Geometry check sheet. Reference: the model listing, model coordinates, mm. A direction names the side the tool comes from. Coordinates: 2 decimals unless noted, no trailing zeros. Write each loop counter-clockwise with the first axis right and the second up, starting at its lowest first coordinate (ties: lowest second). Pieces come first, ordered by that corner, then holes. Notation, with made-up numbers: M 31.5,58 L 72.5,58 A24 ccw 72.5,75 Z; hole C 78,-11 d11. An arc over 180 degrees is marked long. Write item = value, one per line. Start each with the question number.
```python
from build123d import *

# Parameters (mm, degrees)
ESQUISSE3_R             = 35
BOSS_EXTRU_3_DEPTH      = 5
ESQUISSE4_R             = 2
ESQUISSE4_R_2           = 1.6
ENL_V_MAT_EXTRU_1_DEPTH = 161.669919512


with BuildPart() as part:
    # Esquisse3 → Boss.-Extru.3 (new body)
    with BuildSketch(Plane(origin=(0, 0, 0), x_dir=(1, 0, 0), z_dir=(0, 1, 0))):
        with BuildLine():
            Line((-115, -25), (-25, -25))
            Line((-25, -25), (-24.99494949, -24.500051021))
            ThreePointArc((-24.99494949, -24.500051021), (-34.998214236, 0.353553761), (-24.494897428, 25))
            Line((-24.494897428, 25), (-25, 25))
            Line((-25, 25), (-115, 25))
            Line((-115, 25), (-115, -25))
        make_face()
        Circle(ESQUISSE3_R)
        Polygon((-9.403186381, -33.713203436), (35.849364905, -112.092921435), (79.150635095, -87.092921435), (34.150635095, -9.150635095), align=None)
        with BuildLine():
            Line((-24.494897428, 25), (-24.99494949, -24.500051021))
            ThreePointArc((-24.99494949, -24.500051021), (-17.805293657, -30.132565736), (-9.403186381, -33.713203436))
            Line((-9.403186381, -33.713203436), (33.715141323, -9.396235714))
            ThreePointArc((33.715141323, -9.396235714), (34.677297662, -4.741837919), (35, 0))
            ThreePointArc((35, 0), (34.72342821, 4.391302011), (33.898083809, 8.713203436))
            Line((33.898083809, 8.713203436), (-8.720191833, 33.896286735))
            ThreePointArc((-8.720191833, 33.896286735), (-17.19292058, 30.486119496), (-24.494897428, 25))
        make_face()
        Circle(ESQUISSE3_R)
        Polygon((33.898083809, 8.713203436), (79.150635095, 87.092921435), (35.849364905, 112.092921435), (-9.150635095, 34.150635095), align=None)
        with BuildLine():
            ThreePointArc((33.898083809, 8.713203436), (17.805293657, 30.132565736), (-8.720191833, 33.896286735))
            Line((-8.720191833, 33.896286735), (33.898083809, 8.713203436))
        make_face()
    extrude(amount=BOSS_EXTRU_3_DEPTH)

    # Esquisse4 → Enlèv. mat.-Extru.1 (cut, through all)
    with BuildSketch(Plane(origin=(0, 5, 0), x_dir=(1, 0, 0), z_dir=(0, 1, 0))):
        with Locations(Location((-101.75, 20, 0), (0, 0, 270))):
            Circle(ESQUISSE4_R)
        with Locations(Location((-101.75, -20, 0), (0, 0, 270))):
            Circle(ESQUISSE4_R)
        with Locations(Location((33.554491924, -98.118084835, 0), (0, 0, 270))):
            Circle(ESQUISSE4_R)
        with Locations(Location((68.195508076, -78.118084835, 0), (0, 0, 270))):
            Circle(ESQUISSE4_R)
        with Locations(Location((68.195508076, 78.118084835, 0), (0, 0, 270))):
            Circle(ESQUISSE4_R)
        with Locations(Location((33.554491924, 98.118084835, 0), (0, 0, 270))):
            Circle(ESQUISSE4_R)
        with Locations(Location((-3.248264889, -30.973840175, 0), (0, 0, 270))):
            Circle(ESQUISSE4_R_2)
        with Locations(Location((15.051735111, -62.670369954, 0), (0, 0, 270))):
            Circle(ESQUISSE4_R_2)
        with Locations(Location((28.448264889, -12.673840175, 0), (0, 0, 270))):
            Circle(ESQUISSE4_R_2)
        with Locations(Location((46.748264889, -44.370369954, 0), (0, 0, 270))):
            Circle(ESQUISSE4_R_2)
        with Locations(Location((28.448264889, 12.673840175, 0), (0, 0, 270))):
            Circle(ESQUISSE4_R_2)
        with Locations(Location((46.748264889, 44.370369954, 0), (0, 0, 270))):
            Circle(ESQUISSE4_R_2)
        with Locations(Location((15.051735111, 62.670369954, 0), (0, 0, 270))):
            Circle(ESQUISSE4_R_2)
        with Locations(Location((-3.248264889, 30.973840175, 0), (0, 0, 270))):
            Circle(ESQUISSE4_R_2)
        with Locations(Location((-25.2, 18.3, 0), (0, 0, 270))):
            Circle(ESQUISSE4_R_2)
        with Locations(Location((-61.8, -18.3, 0), (0, 0, 270))):
            Circle(ESQUISSE4_R_2)
        with Locations(Location((-25.2, -18.3, 0), (0, 0, 270))):
            Circle(ESQUISSE4_R_2)
        with Locations(Location((-61.8, 18.3, 0), (0, 0, 270))):
            Circle(ESQUISSE4_R_2)
    extrude(amount=-ENL_V_MAT_EXTRU_1_DEPTH, mode=Mode.SUBTRACT)


solid = part.part
```
Q1. Cross-section at B-B on x = -85. Enter the section's corners in (y, z).
Q2. Set-up check for faces 1 (the face through (56.208, 2.465, -47.354)), 2 (the face through (-69, 2, -25)), 3 (the face through (-71, 2, 25)): record each of +Z, -Z, +X, -X, +Y, -Y from which the full face is reachable in a straight line by a thin tool's end or side.
Q3. Cross-section at C-C on z = -38. Enter the section's corners in (x, y), and give its area (3 significant figures).
Q4. Cross-section at A-A on y = 4.05. Count the separate pieces of the cut face and the enclosed holes in it, and give its area (3 significant figures).
Q5. Gauge pin test, flat ends, axial feed: pin 1 (6.5 mm diameter, centred on x = -101.75, z = -20, fed in from -Y); pin 2 (1 mm diameter, centred on y = 4, z = 64, fed in from +X); pin 3 (1 mm diameter, centred on y = 4, z = -56.5, fed in from -X). Record the tip position at first contact, or that the pin passes through.
Q6. Scan lines: L1, parallel to Z at x = -3, y = 2.35; L2, parallel to Z at x = 68, y = 1.35; L3, parallel to Z at x = -59, y = 1.5. Record each from-to range of solid material in increasing order.
Values found:
q1.outline = M 0,-25 L 5,-25 L 5,25 L 0,25 Z
q2.face_1 = +X, +Y, -Y
q2.face_2 = -Z, -X, +Y, -Y
q2.face_3 = +Z, -X, +Y, -Y
q3.outline = M -6.93,0 L 50.81,0 L 50.81,5 L -6.93,5 Z
q3.area = 289 mm²
q4.separate_pieces = 1
q4.enclosed_holes = 18
q4.area = 16,200 mm²
q5.pin_1 = 0
q5.pin_2 = 66.11
q5.pin_3 = 3.46
q6.L1 = -44.8 to -32.55, -29.39 to 29.39, 32.55 to 44.8
q6.L2 = -93.53 to -80.11, -76.13 to -67.78, 67.78 to 76.13, 80.11 to 93.53
q6.L3 = -25 to 25
